```python
from build123d import *

# Parameters (mm, degrees)
SKETCH1_W           = 126
SKETCH1_H           = 71
BOSS_EXTRUDE1_DEPTH = 46
SKETCH2_W           = 20
SKETCH2_H           = 20.5
BOSS_EXTRUDE2_DEPTH = 3
SKETCH3_W           = 120.7
SKETCH3_H           = 66
CUT_EXTRUDE1_DEPTH  = 43
CUT_EXTRUDE2_REACH  = 147.355
CUT_EXTRUDE3_REACH  = 147.355
SKETCH5_W           = 6
SKETCH5_H           = 4
SKETCH6_W           = 6
SKETCH6_H           = 4
CUT_EXTRUDE4_DEPTH  = 121.238305045
CUT_EXTRUDE5_REACH  = 122.238
SKETCH8_R           = 2.4
CUT_EXTRUDE6_DEPTH  = 95.625577937
FILLET1_R           = 3
FILLET2_R           = 4
FILLET3_R           = 2
SKETCH9_R           = 4.5
BOSS_EXTRUDE3_DEPTH = 2.1
SKETCH10_R          = 1.5
CUT_EXTRUDE7_DEPTH  = 94.689967446


with BuildPart() as part:
    # Sketch1 → Boss-Extrude1 (new body)
    with BuildSketch(Plane(origin=(0, 0, 0), x_dir=(1, 0, 0), z_dir=(0, 1, 0))):
        Rectangle(SKETCH1_W, SKETCH1_H)
    extrude(amount=BOSS_EXTRUDE1_DEPTH)

    # Sketch2 → Boss-Extrude2 (add)
    with BuildSketch(Plane.XZ):
        with Locations((-46.5, -45.75)):
            Rectangle(SKETCH2_W, SKETCH2_H)
        with Locations((46.5, -45.75)):
            Rectangle(SKETCH2_W, SKETCH2_H)
    extrude(amount=-BOSS_EXTRUDE2_DEPTH)

    # Sketch3 → Cut-Extrude1 (cut)
    with BuildSketch(Plane(origin=(0, 46, 0), x_dir=(1, 0, 0), z_dir=(0, 1, 0))):
        with Locations((-0.15, 0)):
            Rectangle(SKETCH3_W, SKETCH3_H)
    extrude(amount=-CUT_EXTRUDE1_DEPTH, mode=Mode.SUBTRACT)

    # Sketch4 → Cut-Extrude2 (cut, up to next)
    with BuildSketch(Plane.ZY.offset(63), mode=Mode.PRIVATE) as cut_extrude2_sk1:
        with BuildLine():
            Line((-33, 46), (33, 46))
            Line((33, 46), (33, 18))
            ThreePointArc((33, 18), (28.606601718, 7.393398282), (18, 3))
            Line((18, 3), (-18, 3))
            ThreePointArc((-18, 3), (-28.606601718, 7.393398282), (-33, 18))
            Line((-33, 18), (-33, 46))
        make_face()
    cut_extrude2_tool1 = extrude(cut_extrude2_sk1.sketch, amount=-CUT_EXTRUDE2_REACH, mode=Mode.PRIVATE) & part.part
    add(cut_extrude2_tool1.solids().sort_by_distance((-63, 25.139342, 0))[0], mode=Mode.SUBTRACT)

    # Sketch5 → Cut-Extrude3 (cut, up to next)
    with BuildSketch(Plane(origin=(63, 0, 0), x_dir=(0, 0, -1), z_dir=(1, 0, 0)), mode=Mode.PRIVATE) as cut_extrude3_sk1:
        with BuildLine():
            Line((-16.5, 46), (16.5, 46))
            Line((16.5, 46), (16.5, 42.8))
            ThreePointArc((16.5, 42.8), (15.09411255, 39.40588745), (11.7, 38))
            Line((11.7, 38), (-11.7, 38))
            ThreePointArc((-11.7, 38), (-15.09411255, 39.40588745), (-16.5, 42.8))
            Line((-16.5, 42.8), (-16.5, 46))
        make_face()
    cut_extrude3_tool1 = extrude(cut_extrude3_sk1.sketch, amount=-CUT_EXTRUDE3_REACH, mode=Mode.PRIVATE) & part.part
    # Sketch5 → Cut-Extrude3 (cut, up to next)
    with BuildSketch(Plane(origin=(63, 0, 0), x_dir=(0, 0, -1), z_dir=(1, 0, 0)), mode=Mode.PRIVATE) as cut_extrude3_sk2:
        with Locations((22.5, 42)):
            Rectangle(SKETCH5_W, SKETCH5_H)
    cut_extrude3_tool2 = extrude(cut_extrude3_sk2.sketch, amount=-CUT_EXTRUDE3_REACH, mode=Mode.PRIVATE) & part.part
    # Sketch5 → Cut-Extrude3 (cut, up to next)
    with BuildSketch(Plane(origin=(63, 0, 0), x_dir=(0, 0, -1), z_dir=(1, 0, 0)), mode=Mode.PRIVATE) as cut_extrude3_sk3:
        with Locations((-22.5, 42)):
            Rectangle(SKETCH5_W, SKETCH5_H)
    cut_extrude3_tool3 = extrude(cut_extrude3_sk3.sketch, amount=-CUT_EXTRUDE3_REACH, mode=Mode.PRIVATE) & part.part
    add(cut_extrude3_tool1.solids().sort_by_distance((63, 42.113938, 0))[0], mode=Mode.SUBTRACT)
    add(cut_extrude3_tool2.solids().sort_by_distance((63, 42, -22.5))[0], mode=Mode.SUBTRACT)
    add(cut_extrude3_tool3.solids().sort_by_distance((63, 42, 22.5))[0], mode=Mode.SUBTRACT)

    # Sketch6 → Cut-Extrude4 (cut, through all)
    with BuildSketch(Plane.XY.offset(35.5)):
        with Locations((-54.5, 42)):
            Rectangle(SKETCH6_W, SKETCH6_H)
    extrude(amount=-CUT_EXTRUDE4_DEPTH, mode=Mode.SUBTRACT)

    # Sketch7 → Cut-Extrude5 (cut, up to next)
    with BuildSketch(Plane.XY.offset(35.5), mode=Mode.PRIVATE) as cut_extrude5_sk1:
        with BuildLine():
            Line((-27.7, 28.2), (-22.1, 28.2))
            ThreePointArc((-22.1, 28.2), (-19.766547622, 27.233452378), (-18.8, 24.9))
            Line((-18.8, 24.9), (-18.8, 24.3))
            ThreePointArc((-18.8, 24.3), (-19.766547622, 21.966547622), (-22.1, 21))
            Line((-22.1, 21), (-27.7, 21))
            ThreePointArc((-27.7, 21), (-30.033452378, 21.966547622), (-31, 24.3))
            Line((-31, 24.3), (-31, 24.9))
            ThreePointArc((-31, 24.9), (-30.033452378, 27.233452378), (-27.7, 28.2))
        make_face()
    cut_extrude5_tool1 = extrude(cut_extrude5_sk1.sketch, amount=-CUT_EXTRUDE5_REACH, mode=Mode.PRIVATE) & part.part
    add(cut_extrude5_tool1.solids().sort_by_distance((-24.9, 24.6, 35.5))[0], mode=Mode.SUBTRACT)

    # Sketch8 → Cut-Extrude6 (cut, through all)
    with BuildSketch(Plane(origin=(0, 3, 0), x_dir=(1, 0, 0), z_dir=(0, 1, 0))):
        with Locations(Location((-46.5, 46, 0), (0, 0, 270))):
            Circle(SKETCH8_R)
        with Locations(Location((46.5, 46, 0), (0, 0, 270))):
            Circle(SKETCH8_R)
    extrude(amount=-CUT_EXTRUDE6_DEPTH, mode=Mode.SUBTRACT)

    # Fillet1
    fillet1_edges = [part.edges().sort_by_distance(p)[0] for p in [
        (36.5, 1.5, -56),
        (56.5, 1.5, -56),
        (-36.5, 1.5, -56),
        (-56.5, 1.5, -56),
    ]]
    fillet(fillet1_edges, radius=FILLET1_R)

    # Fillet2
    fillet2_edges = [part.edges().sort_by_distance(p)[0] for p in [
        (-56.5, 1.5, -35.5),
        (-36.5, 1.5, -35.5),
        (56.5, 1.5, -35.5),
        (36.5, 1.5, -35.5),
    ]]
    fillet(fillet2_edges, radius=FILLET2_R)

    # Fillet3
    fillet3_edges = [part.edges().sort_by_distance(p)[0] for p in [
        (-46.5, 0, -56),
        (-36.5, 0, -46.25),
        (46.5, 0, -56),
        (56.5, 0, -46.25),
        (-55.621320344, 0, -55.121320344),
        (-37.378679656, 0, -55.121320344),
        (55.621320344, 0, -55.121320344),
        (37.378679656, 0, -55.121320344),
        (0, 0, -35.5),
        (-61.75, 0, -35.5),
        (-56.5, 0, -46.25),
        (36.5, 0, -46.25),
        (-57.671572875, 0, -36.671572875),
        (-35.328427125, 0, -36.671572875),
        (57.671572875, 0, -36.671572875),
        (35.328427125, 0, -36.671572875),
        (0, 0, 35.5),
        (-63, 0, 0),
        (61.75, 0, -35.5),
        (63, 0, 0),
        (63, 23, 35.5),
        (-63, 23, 35.5),
        (-63, 23, -35.5),
        (63, 23, -35.5),
    ]]
    fillet(fillet3_edges, radius=FILLET3_R)

    # Sketch9 → Boss-Extrude3 (add)
    with BuildSketch(Plane(origin=(0, 3, 0), x_dir=(1, 0, 0), z_dir=(0, 1, 0))):
        with Locations(Location((-45, 28, 0), (0, 0, 270))):
            Circle(SKETCH9_R)
        with Locations(Location((-46.4, -20.3, 0), (0, 0, 270))):
            Circle(SKETCH9_R)
        with Locations(Location((31, 18, 0), (0, 0, 270))):
            Circle(SKETCH9_R)
        with Locations(Location((36.6, -20.3, 0), (0, 0, 270))):
            Circle(SKETCH9_R)
    extrude(amount=BOSS_EXTRUDE3_DEPTH)

    # Sketch10 → Cut-Extrude7 (cut, through all)
    with BuildSketch(Plane(origin=(0, 5.1, 0), x_dir=(1, 0, 0), z_dir=(0, 1, 0))):
        with Locations(Location((-45, 28, 0), (0, 0, 270))):
            Circle(SKETCH10_R)
        with Locations(Location((-46.4, -20.3, 0), (0, 0, 270))):
            Circle(SKETCH10_R)
        with Locations(Location((36.6, -20.3, 0), (0, 0, 270))):
            Circle(SKETCH10_R)
    extrude(amount=-CUT_EXTRUDE7_DEPTH, mode=Mode.SUBTRACT)


solid = part.part
```
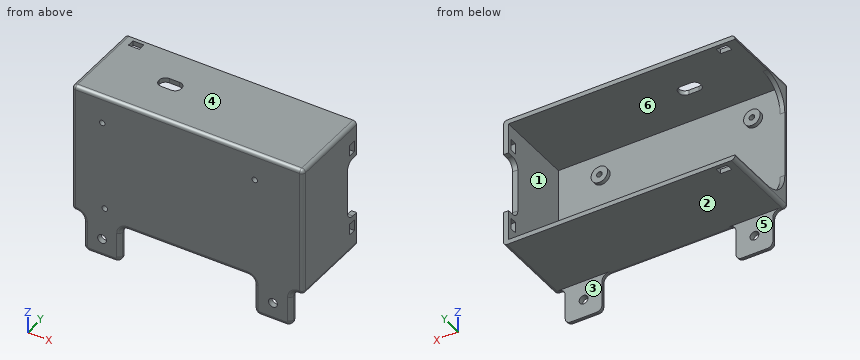
Check sheet for the modelled part. Datum: model origin and axes. Units: mm. Face numbers are marked on the shaded views. A direction names the side the tool comes from. Coordinates: 2 decimals unless noted, no trailing zeros. Loops run counter-clockwise (first coordinate to the right, second up) from the corner with the lowest first, then second, coordinate; pieces in that order, holes last. Notation, with made-up numbers: M 10.5,54 L 33.5,54 A19 cw 33.5,79 Z; hole C 89,25 d10. An arc over 180 degrees is marked long. Answer as a JSON object with one key per item and string values.
1. Sectioned sample at A-A on z = 30. Record the cut outline in (x, y), and give its area (3 significant figures).
Outcome:
{"outline": "M -63,2 A2 ccw -61,0 L 61,0 A2 ccw 63,2 L 63,46 L 60.2,46 L 60.2,3 L -60.5,3 L -60.5,9 L -63,9 Z", "area": "512 mm²"}
2. Sectioned sample at C-C on z = -28. Record the cut outline in (x, y).
Outcome:
{"outline": "M -63,2 A2 ccw -61,0 L -46.5,0 L -46.5,5.1 L -49.5,5.1 L -49.5,3 L -60.5,3 L -60.5,6.82 L -63,6.82 Z; M -43.5,0 L 61,0 A2 ccw 63,2 L 63,46 L 60.2,46 L 60.2,3 L -40.5,3 L -40.5,5.1 L -43.5,5.1 Z"}
3. Depth check by flat-ended pin: P1, Ø0.5, axis at y = 2.5, z = -49.5, coming from the +X side; P2, Ø22.5, axis at x = -49, z = -46.5, coming from the +Y side; P3, Ø1.1, axis at y = 2.5, z = -48.5, coming from the -X side; P4, Ø21.5, axis at x = 7, y = 26, coming from the -Z side. Enter the tip coordinate at first touch or a pass-through.
Outcome:
{"P1": "x = 56.5", "P2": "y = 46", "P3": "x = -56.5", "P4": "z = -35.5"}
4. Release check for a two-part mould opening along Z. For the marked faces 1, 2 and 3 record: pulls with the +Z half, pulls with the -Z half, needs draft (parallel to the pull), parting line crosses it, or undercut.
Outcome:
{"face 1": "undercut", "face 2": "pulls with the -Z half", "face 3": "needs draft"}
5. Access from +Z, -Z, +X, -X, +Y, -Y to the whole of each face (thin tool, end or side, straight path). Record for the marked faces 4, 5 and 6.
Outcome:
{"face 4": "+Z, +X, -X, +Y, -Y", "face 5": "-Z, +X, -X, +Y", "face 6": "+Y"}
6. Scan lines: L1, parallel to X at y = 2.95, z = 20.3; L2, parallel to Z at x = -41, y = 35; L3, parallel to X at y = 2.3, z = -46. Record each from-to range of solid material in increasing order. Write a range as from..to.
Outcome:
{"L1": "-63..-47.9, -44.9..35.1, 38.1..63", "L2": "-35.5..-33, 33..35.5", "L3": "-56.5..-48.9, -44.1..-36.5, 36.5..44.1, 48.9..56.5"}
7. Sectioned sample at D-D on z = -9.5. Record the cut outline in (x, y).
Outcome:
{"outline": "M -63,2 A2 ccw -61,0 L 61,0 A2 ccw 63,2 L 63,38 L 60.2,38 L 60.2,3 L -63,3 Z"}
8. Sectioned sample at B-B on x = -7.5. Record the cut outline in (y, z).
Outcome:
{"outline": "M 0,-33.5 A2 ccw 2,-35.5 L 46,-35.5 L 46,-33 L 3,-33 L 3,33 L 46,33 L 46,35.5 L 2,35.5 A2 ccw 0,33.5 Z"}
